CAD build for the part. Positions are in the model's coordinates, mm. Face numbers are marked on the shaded views. Coordinates: 2 decimals unless noted, no trailing zeros. Write each loop counter-clockwise with the first axis right and the second up, starting at its lowest first coordinate (ties: lowest second). Pieces come first, ordered by that corner, then holes.
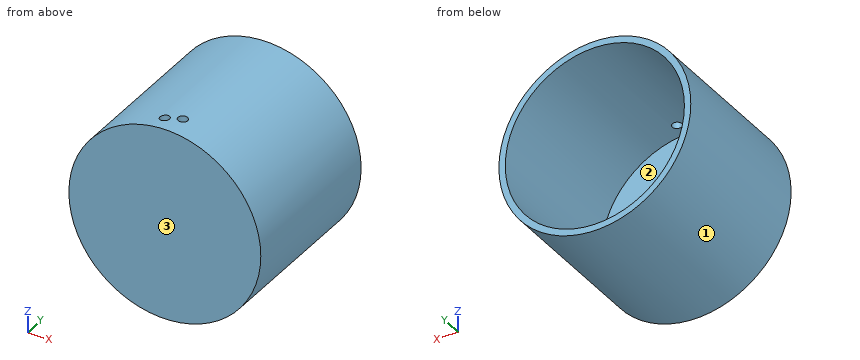
Autodesk Inventor part; units mm, degrees
ref_plane "Work Plane1" through (0, 0, 30) normal (0, 0, 1) x (1, 0, 0)
ref_plane "YZ Plane" through (0, 0, 0) normal (1, 0, 0) x (0, 1, 0)
ref_plane "XZ Plane" through (0, 0, 0) normal (0, 1, 0) x (-1, 0, 0)
sketch "Sketch1" plane through (0, 0, 0) normal (0, 1, 0) x (-1, 0, 0)
  circle A0 centre (0, 0) radius 30
  dimension "d0" = 60
extrude "Extrusion1" add sketch "Sketch1" along normal blind 50.8
shell "Shell1" thickness 2 removed faces 1 at (-9.4188, 50.8, 0)
ref_plane "Work Plane1" through (0, 0, 30) normal (0, 0, 1) x (1, 0, 0)
sketch "Sketch2" plane through (0, 0, 30) normal (0, 0, 1) x (1, 0, 0)
  line L0 (28, 2) -> (-28, 2)
  circle A0 centre (-3.1214, 5) radius 1.5
  circle A1 centre (1.3586, 6.9) radius 1.5
  point P0 (0, 0)
  dimension "d4" = 3
  dimension "d5" = 3
  dimension "d6" = 4.48
  dimension "d7" = 1.9
  dimension "d8" = 3
extrude "Extrusion2" cut sketch "Sketch2" against normal blind 4
properties part number "Simple Pressure Gauge Cup 23-02-03"
Item 1: Wall check: line 1 along Y through (x, z) = (2, 9.5); line 2 along X through (y, z) = (13.5, -18); line 3 along X through (y, z) = (37, -10). Give the ranges that are in metal, low to high.
Item 2: Saw through at A-A, the plane x = -3.5. Write the cut outline in (y, z).
Item 3: Saw through at B-B, the plane z = 0. Write the cut outline in (x, y), and give its area (3 significant figures).
Item 4: Two-plate mould, pull along Z, no slides. Class the marked faces 1, 2 and 3: +Z half, -Z half, draft (parallel to the pull), parting line (faces both ways), or undercut.
Item 5: Saw through at C-C, the plane y = 43. Write the cut outline in (x, z).
Item 6: Saw through at D-D, the plane x = -20.5. Write the cut outline in (y, z), and give its area (3 significant figures).
Item 7: Flat gauge pins, fed straight in: pin 1 Ø4 at (x, y) = (-13, 38.5) entering from -Z; pin 2 Ø4 at (x, y) = (-21, 44) entering from +Z; pin 3 Ø6 at (x, z) = (8.5, -19) entering from +Y. Where does each tip first touch, or does it go through?
Working result:
1. line 1: y = 0 to 2
1. line 2: x = -24 to -21.45, 21.45 to 24
1. line 3: x = -28.28 to -26.15, 26.15 to 28.28
2. outline: (0, -29.8) - (50.8, -29.8) - (50.8, -27.78) - (2, -27.78) - (2, 27.78) - (3.55, 27.78) - (3.55, 29.8) - (0, 29.8) - close; (6.45, 27.78) - (50.8, 27.78) - (50.8, 29.8) - (6.45, 29.8) - close
3. outline: (-30, 0) - (30, 0) - (30, 50.8) - (28, 50.8) - (28, 2) - (-28, 2) - (-28, 50.8) - (-30, 50.8) - close
3. area: 315 mm2
4. face 1: parting line
4. face 2: undercut
4. face 3: draft
5. outline: circle Ø60 at (0, 0); hole circle Ø56 at (0, 0)
6. outline: (0, -21.9) - (50.8, -21.9) - (50.8, -19.07) - (2, -19.07) - (2, 19.07) - (50.8, 19.07) - (50.8, 21.9) - (0, 21.9) - close
6. area: 364 mm2
7. pin 1: stops at z = -27.91
7. pin 2: stops at z = 23.22
7. pin 3: stops at y = 2
